Can you work these out from the model? Positions are in its coordinate system, mm. A direction names the side the tool comes from. Coordinates: 2 decimals unless noted, no trailing zeros. Order: outer loops, then holes, each group sorted by start corner. A loop starts at its lowest first (then second) coordinate and runs counter-clockwise, first axis right, second up. Notation, with made-up numbers: (57.25, -34) - (98.25, -34) arc R21 ccw to (98.25, -2) - close; hole circle Ø4 at (-32.5, 55.25). An arc over 180 degrees is marked (long way). Use a Markdown table: item, result. Add a question column.
(1) I want a section at B-B (x = -40). List the corners of the cut face in (y, z) for me, and give its area (4 significant figures).
(2) We'd pull the mould along Y, two halves only. Please class faces 1 (the flat face through (-5, 4.762, 1)), 2 (the flat face through (-68.36, -0.07, 1.1)), 3 (the conical face through (-52.855, -0.655, 0.986)): pulls with the +Y half, pulls with the -Y half, needs draft (parallel to the pull), parting line crosses it, or undercut.
(3) On a 3-axis mill with a long thin cutter (end or side, diameter ignored), from which of +Z, -Z, +X, -X, +Y, -Y can I reach the whole of each face in a straight line? I mean faces 4 (the flat face through (0, -1, 2)), 5 (the cylindrical face through (-76.655, -5.27, 0.108)), 6 (the flat face through (62.5, -0.1, -1.3)). Say none if no direction works.
(4) I want a section at A-A (y = 0). List the corners of the cut face in (x, z) for me (3 decimals).
(5) For pin 1 Ø5.5 at (x, y) = (-10, -1) entering from +Z; pin 2 Ø2 at (y, z) = (-1, 3) entering from -X; pin 3 Ø0.5 at (x, y) = (21, -5.5) entering from -Z, each with a flat end and sliding along its axis, tell me the tip position at first contact or that it passes through.
(6) If I drill on L1, parallel to Z at x = -16.5, y = -2; L2, parallel to Y at x = -25, z = -2.25; L3, parallel to Y at x = 20, z = 1.75, over which ranges is the centre line in solid material (lowest first)? Write a range as [from, to].
```python
from build123d import *

# Parameters (mm, degrees)
EXTRUDE_THIN1_DEPTH          = 9.525
SKETCH3_R                    = 1.65
CUT_EXTRUDE1_DEPTH           = 75.946970354
CUT_EXTRUDE1_DRAFT           = 3.5
CUT_EXTRUDE1_PROFILE_2_DEPTH = 75.946970354
CUT_EXTRUDE1_PROFILE_2_DRAFT = 3.5
CUT_EXTRUDE1_PROFILE_3_DEPTH = 75.946970354
CUT_EXTRUDE1_PROFILE_3_DRAFT = 3.5
EXTRUDE_THIN2_START          = 1
EXTRUDE_THIN2_DEPTH          = 1


with BuildPart() as part:
    # Sketch2 → Extrude-Thin1 (new body)
    with BuildSketch(Plane.XZ.offset(4.7625)):
        with BuildLine():
            Line((63.25, -2.598076211), (61.75, 0))
            Line((61.75, 0), (-64.275, 0))
            Line((-64.275, 0), (-72.561586906, 2.235175454))
            ThreePointArc((-72.561586906, 2.235175454), (-73.854260092, 2.964003531), (-74.639461328, 4.223230813))
            Line((-74.639461328, 4.223230813), (-72.733358502, 4.828847868))
            ThreePointArc((-72.733358502, 4.828847868), (-72.471624756, 4.409105441), (-72.040733695, 4.166162748))
            Line((-72.040733695, 4.166162748), (-64.010001325, 2))
            Line((-64.010001325, 2), (62.904700538, 2))
            Line((62.904700538, 2), (64.982050808, -1.598076211))
            Line((64.982050808, -1.598076211), (63.25, -2.598076211))
        make_face()
    extrude(amount=-EXTRUDE_THIN1_DEPTH)


with BuildPart() as cut_extrude1_tool:
    # Sketch3 → Cut-Extrude1 (with draft: the straight prism first)
    with BuildSketch(Plane(origin=(0, 0, 0), x_dir=(-1, 0, 0), z_dir=(0, 0, -1))):
        with Locations((51.275, 0)):
            Circle(SKETCH3_R)
    extrude(amount=-CUT_EXTRUDE1_DEPTH)
    # Cut-Extrude1: the draft: its side faces are tilted about the plane it starts from
    cut_extrude1_sides = [cut_extrude1_tool.faces().sort_by_distance(p)[0] for p in [
        (-49.625, 0, 37.973485177),
    ]]
    draft(cut_extrude1_sides, Plane(origin=(0, 0, 0), x_dir=(-1, 0, 0), z_dir=(0, 0, -1)), CUT_EXTRUDE1_DRAFT)


with BuildPart() as part_1:
    add(part.part)

    # Cut-Extrude1: cut by cut_extrude1_tool
    add(cut_extrude1_tool.part, mode=Mode.SUBTRACT)


with BuildPart() as cut_extrude1_profile_2_tool:
    # Sketch3 → Cut-Extrude1 profile 2 (with draft: the straight prism first)
    with BuildSketch(Plane(origin=(0, 0, 0), x_dir=(-1, 0, 0), z_dir=(0, 0, -1))):
        with Locations((16.275, 0)):
            Circle(SKETCH3_R)
    extrude(amount=-CUT_EXTRUDE1_PROFILE_2_DEPTH)
    # Cut-Extrude1 profile 2: the draft: its side faces are tilted about the plane it starts from
    cut_extrude1_profile_2_sides = [cut_extrude1_profile_2_tool.faces().sort_by_distance(p)[0] for p in [
        (-14.625, 0, 37.973485177),
    ]]
    draft(cut_extrude1_profile_2_sides, Plane(origin=(0, 0, 0), x_dir=(-1, 0, 0), z_dir=(0, 0, -1)), CUT_EXTRUDE1_PROFILE_2_DRAFT)


with BuildPart() as part_2:
    add(part_1.part)

    # Cut-Extrude1 profile 2: cut by cut_extrude1_profile_2_tool
    add(cut_extrude1_profile_2_tool.part, mode=Mode.SUBTRACT)


with BuildPart() as cut_extrude1_profile_3_tool:
    # Sketch3 → Cut-Extrude1 profile 3 (with draft: the straight prism first)
    with BuildSketch(Plane(origin=(0, 0, 0), x_dir=(-1, 0, 0), z_dir=(0, 0, -1))):
        with Locations((-18.725, 0)):
            Circle(SKETCH3_R)
    extrude(amount=-CUT_EXTRUDE1_PROFILE_3_DEPTH)
    # Cut-Extrude1 profile 3: the draft: its side faces are tilted about the plane it starts from
    cut_extrude1_profile_3_sides = [cut_extrude1_profile_3_tool.faces().sort_by_distance(p)[0] for p in [
        (20.375, 0, 37.973485177),
    ]]
    draft(cut_extrude1_profile_3_sides, Plane(origin=(0, 0, 0), x_dir=(-1, 0, 0), z_dir=(0, 0, -1)), CUT_EXTRUDE1_PROFILE_3_DRAFT)


with BuildPart() as part_3:
    add(part_2.part)

    # Cut-Extrude1 profile 3: cut by cut_extrude1_profile_3_tool
    add(cut_extrude1_profile_3_tool.part, mode=Mode.SUBTRACT)

    # Sketch2<2> → Extrude-Thin2 (add)
    with BuildSketch(Plane.XZ.offset(4.7625).offset(EXTRUDE_THIN2_START)):
        with BuildLine():
            Line((64.982050808, -1.598076211), (62.904700538, 2))
            Line((62.904700538, 2), (-64.010001325, 2))
            Line((-64.010001325, 2), (-72.040733695, 4.166162748))
            ThreePointArc((-72.040733695, 4.166162748), (-72.471624756, 4.409105441), (-72.733358502, 4.828847868))
            Line((-72.733358502, 4.828847868), (-78.451666979, 3.011996703))
            ThreePointArc((-78.451666979, 3.011996703), (-76.619530762, 0.073799711), (-73.603293329, -1.626799136))
            Line((-73.603293329, -1.626799136), (-64.804997349, -4))
            Line((-64.804997349, -4), (59.440598923, -4))
            Line((59.440598923, -4), (59.785898385, -4.598076211))
            Line((59.785898385, -4.598076211), (64.982050808, -1.598076211))
        make_face()
    extrude(amount=-EXTRUDE_THIN2_DEPTH)


solid = part_3.part
```
Answers follow:
| question | item | result |
|---|---|---|
| 1 | outline | (-5.76, -4) - (-4.76, -4) - (-4.76, 0) - (4.76, 0) - (4.76, 2) - (-5.76, 2) - close |
| 1 | area | 25.05 mm² |
| 2 | face 1 | pulls with the +Y half |
| 2 | face 2 | needs draft |
| 2 | face 3 | undercut |
| 3 | face 4 | +Z, +X, +Y, -Y |
| 3 | face 5 | -Z, -X, +Y, -Y |
| 3 | face 6 | -Z, -X, +Y |
| 4 | outline | (-74.639, 4.223) arc R3 ccw to (-72.562, 2.235) - (-64.275, 0) - (-52.925, 0) - (-53.047, 2) - (-64.01, 2) - (-72.041, 4.166) arc R1 cw to (-72.733, 4.829) - close; (-49.625, 0) - (-17.925, 0) - (-18.047, 2) - (-49.503, 2) - close; (-14.625, 0) - (17.075, 0) - (16.953, 2) - (-14.503, 2) - close; (20.375, 0) - (61.75, 0) - (63.25, -2.598) - (64.982, -1.598) - (62.905, 2) - (20.497, 2) - close |
| 5 | pin 1 | stops at z = 2 |
| 5 | pin 2 | stops at x = -74.56 |
| 5 | pin 3 | stops at z = -4 |
| 6 | L1 | z = [0, 2] |
| 6 | L2 | y = [-5.76, -4.76] |
| 6 | L3 | y = [-5.76, -1.21], [1.21, 4.76] |
